Autodesk Inventor part; units mm, degrees
ref_plane "YZ Plane" through (0, 0, 0) normal (1, 0, 0) x (0, 1, 0)
ref_plane "XZ Plane" through (0, 0, 0) normal (0, 1, 0) x (-1, 0, 0)
ref_plane "XY Plane" through (0, 0, 0) normal (0, 0, 1) x (1, 0, 0)
sketch "Sketch1" plane through (0, 0, 0) normal (0, 1, 0) x (-1, 0, 0)
  line L0 (0, 0) -> (3, 0)
  line L1 (3, 0) -> (3, -25)
  line L2 (3, -25) -> (0, -25)
  line L3 (0, -25) -> (0, 0)
  line L4 (8.2, 0) -> (11.2, 0)
  line L5 (11.2, 0) -> (11.2, -25)
  line L6 (11.2, -25) -> (8.2, -25)
  line L7 (8.2, -25) -> (8.2, 0)
  point P0 (0, -12.5)
  point P1 (8.2, -12.5)
  dimension "d0" = 25
  dimension "d1" = 3
  dimension "d2" = 25
  dimension "d3" = 3
  dimension "d4" = 5.2
extrude "Extrusion1" add sketch "Sketch1" along normal blind 15
sketch "Sketch2" plane through (0, 15, 0) normal (0, 1, 0) x (1, 0, 0)
  line L0 (-11.2, 25) -> (-11.2, 0)
  line L1 (-11.2, 0) -> (0, 0)
  line L2 (0, 0) -> (0, 25)
  line L3 (0, 25) -> (-11.2, 25)
  line L4 (-11.2, 25) -> (-11.2, 0)
  point P0 (0, 0)
extrude "Extrusion2" add sketch "Sketch2" along normal blind 10
sketch "Sketch3" plane through (0, 0, 0) normal (1, 0, 0) x (0, 0, -1)
  line L0 (0, 25) -> (25, 25)
  line L1 (12.5, 25) -> (12.5, 0.2306)
  line L2 (9.5, 25) -> (9.5, 21)
  line L3 (9.5, 21) -> (7.8272, 21)
  line L4 (7.8272, 21) -> (7.8272, 16)
  line L5 (7.8272, 16) -> (12.5, 16)
  line L6 (15.5, 25) -> (15.5, 21)
  line L7 (15.5, 21) -> (17.1728, 21)
  line L8 (17.1728, 21) -> (17.1728, 16)
  line L9 (17.1728, 16) -> (12.5, 16)
  line L10 (9.5, 25) -> (15.5, 25)
  circle A0 centre (12.5, 3.7087) radius 2.6
  point P0 (0, 0)
  point P1 (8.6636, 21)
  dimension "d9" = 6
  dimension "d10" = 5
  dimension "d11" = 8
  dimension "d14" = 5.2
extrude "Extrusion3" cut sketch "Sketch3" against normal blind 20
sketch "Sketch4" plane through (0, 0, 0) normal (1, 0, 0) x (0, 0, -1)
  line L0 (0, 0) -> (25, 0)
  line L1 (25, 0) -> (25, 25)
  line L2 (0, 0) -> (25, 0)
  line L3 (25, 0) -> (25, 20.8379)
  line L4 (25, 20.8379) -> (0, 20.8379)
  line L5 (0, 20.8379) -> (0, 0)
extrude "Extrusion4" cut sketch "Sketch4" against normal blind 8.25
properties part number "RollXAxisEnd" material "Thermoplastic Resin"
CAD build for the part. Positions are in the model's coordinates, mm. A direction names the side the tool comes from. Round coordinates to 2 decimals unless told otherwise and drop trailing zeros. Order: outer loops, then holes, each group sorted by start corner. A loop starts at its lowest first (then second) coordinate and runs counter-clockwise, first axis right, second up.
Q1. Slice it at B-B (z = -12.5). Write the cut outline in (x, y).
Q2. Wall check: L1, parallel to Y at x = -8.5, z = -8.75; L2, parallel to Y at x = -9.5, z = -12.5; L3, parallel to Y at x = -3, z = -16.5. Give the ranges that are in metal, low to high.
Q3. Drop flat-ended pins along their axis: pin 1 (6.5 mm diameter, centred on y = 12, z = -9.5, fed in from +X); pin 2 (6.5 mm diameter, centred on x = -3, z = -5.5, fed in from -Y); pin 3 (0.9 mm diameter, centred on x = -9.5, z = -14.5, fed in from +Y); pin 4 (4 mm diameter, centred on x = -4, y = 18.5, fed in from +Z). Give the stop position or say it passes through.
Q4. Slice it at C-C (y = 3). Write the cut outline in (x, z).
Q5. Slice it at D-D (y = 10). Write the cut outline in (x, z).
Q6. Two-plate mould, pull along Z, no slides. Class faces 1 (the flat face through (-10, 16, -12)), 2 (the flat face through (-11.2, 12, -13)), 3 (the flat face through (-8.5, 15.2, -25)), 4 (the flat face through (-9, 19, -7.827)): pulls with the +Z half, pulls with the -Z half, needs draft (parallel to the pull), parting line crosses it, or undercut.
Q7. Slice it at A-A (x = -1.75). Write the cut outline in (y, z), and give its area (3 significant figures).
Q8. Which spindle directions (+Z, -Z, +X, -X, +Y, -Y) get a long thin tool onto all of the face, cutting with end or side? Do faces 5 (the flat face through (-4, 20.838, -4)), 6 (the flat face through (-6, 25, -5)), 7 (the flat face through (-9, 19, -17.173)), 8 (the flat face through (-6, 23, -15.5)), 9 (the flat face through (-9, 16, 0)). Say none if no direction does.
Results below:
1. outline: (-11.2, 0) - (-8.25, 0) - (-8.25, 1.11) - (-11.2, 1.11) - close; (-11.2, 6.31) - (-8.25, 6.31) - (-8.25, 16) - (-11.2, 16) - close
2. L1: y = 0 to 16, 21 to 25
2. L2: y = 0 to 1.11, 6.31 to 16
2. L3: y = 21 to 25
3. pin 1: stops at x = -8.25
3. pin 2: stops at y = 20.84
3. pin 3: stops at y = 16
3. pin 4: passes through
4. outline: (-11.2, -25) - (-8.25, -25) - (-8.25, -15) - (-11.2, -15) - close; (-11.2, -10) - (-8.25, -10) - (-8.25, 0) - (-11.2, 0) - close
5. outline: (-11.2, -25) - (-8.25, -25) - (-8.25, 0) - (-11.2, 0) - close
6. face 1: undercut
6. face 2: needs draft
6. face 3: pulls with the -Z half
6. face 4: undercut
7. outline: (20.84, -25) - (25, -25) - (25, -15.5) - (21, -15.5) - (21, -17.17) - (20.84, -17.17) - close; (20.84, -7.83) - (21, -7.83) - (21, -9.5) - (25, -9.5) - (25, 0) - (20.84, 0) - close
7. area: 78.5 mm2
8. face 5: +Z, -Z, +X, -Y
8. face 6: +Z, -Z, +X, -X, +Y
8. face 7: +X, -X
8. face 8: +X, -X, +Y
8. face 9: +Z, +X, -X, +Y, -Y
